```python
from build123d import *

# Parameters (mm, degrees)
SKETCH1_W           = 215
SKETCH1_H           = 14
BOSS_EXTRUDE1_DEPTH = 2
SKETCH2_W           = 215
SKETCH2_H           = 2
BOSS_EXTRUDE2_DEPTH = 4
SKETCH3_W           = 10
SKETCH3_H           = 10
BOSS_EXTRUDE3_DEPTH = 2
CUT_EXTRUDE1_DEPTH  = 4
BOSS_EXTRUDE4_START = -175
SKETCH8_W           = 10
SKETCH8_H           = 10
BOSS_EXTRUDE4_DEPTH = 50
CUT_EXTRUDE5_DEPTH  = 50
FILLET2_R           = 10
CUT_EXTRUDE6_DEPTH  = 10


with BuildPart() as part:
    # Sketch1 → Boss-Extrude1 (new body)
    with BuildSketch(Plane.XY):
        with Locations((-78.55, 1.825)):
            Rectangle(SKETCH1_W, SKETCH1_H)
    extrude(amount=BOSS_EXTRUDE1_DEPTH)

    # Sketch2 → Boss-Extrude2 (add)
    with BuildSketch(Plane.XY.offset(2)):
        with Locations((-78.55, -4.175)):
            Rectangle(SKETCH2_W, SKETCH2_H)
    extrude(amount=BOSS_EXTRUDE2_DEPTH)

    # Sketch3 → Boss-Extrude3 (add)
    with BuildSketch(Plane(origin=(0, 0, 0), x_dir=(-1, 0, 0), z_dir=(0, 0, -1))):
        with Locations((-33.95, 3.825)):
            Rectangle(SKETCH3_W, SKETCH3_H)
    extrude(amount=-BOSS_EXTRUDE3_DEPTH)

    # Sketch4 → Cut-Extrude1 (cut)
    with BuildSketch(Plane.XY.offset(6)):
        Polygon((28.95, -5.175), (8.95, -5.175), (3.95, -3.175), (28.95, -3.175), align=None)
    extrude(amount=-CUT_EXTRUDE1_DEPTH, mode=Mode.SUBTRACT)

    # Sketch8 → Boss-Extrude4 (add)
    with BuildSketch(Plane.ZY.offset(186.05).offset(BOSS_EXTRUDE4_START)):
        with Locations((7, 3.825)):
            Rectangle(SKETCH8_W, SKETCH8_H)
    extrude(amount=-BOSS_EXTRUDE4_DEPTH)

    # Sketch12 → Cut-Extrude5 (cut)
    with BuildSketch(Plane.XZ.offset(1.175)):
        Polygon((38.95, 0), (34.10168529, 12), (38.95, 12), align=None)
    extrude(amount=-CUT_EXTRUDE5_DEPTH, mode=Mode.SUBTRACT)

    # Fillet2
    fillet2_edges = [part.edges().sort_by_distance(p)[0] for p in [
        (36.525842645, 8.825, 6),
    ]]
    fillet(fillet2_edges, radius=FILLET2_R - 0.0001)  # a hair under: the kernel refuses the full size

    # Sketch13 → Cut-Extrude6 (cut)
    with BuildSketch(Plane.XY.offset(12)):
        with BuildLine():
            Line((-11.05, 8.825), (-11.05, -1.175))
            Line((-11.05, -1.175), (34.10168529, -1.175))
            add(Edge.make_bspline(
                [(-11.05, 8.825), (3.606248202, 7.334330419), (22.993995007, 11.334895317), (34.10168529, -1.175)],
                knots=[0, 0, 0, 0, 1, 1, 1, 1], degree=3))
        make_face()
    extrude(amount=-CUT_EXTRUDE6_DEPTH, mode=Mode.SUBTRACT)


solid = part.part
```
Verification items for the finished model (mm, model axes). A direction names the side the tool comes from. Coordinates: 2 decimals unless noted, no trailing zeros. Write each loop counter-clockwise with the first axis right and the second up, starting at its lowest first coordinate (ties: lowest second). Pieces come first, ordered by that corner, then holes. Notation, with made-up numbers: M 10.5,16 L 35.5,16 A22 cw 35.5,43 Z; hole C 6,-32 d2. An arc over 180 degrees is marked long. Answer as a JSON object with one key per item and string values. Group by question number.
(1) Cross-section at A-A, the plane x = -72.5. Record the cut outline in (y, z) (3 decimals), and give its area (3 significant figures).
(2) Tool access check on faces 1 (the face through (-30, 8.825, 1)), 2 (the face through (6.485, -4.189, 4.028)), 3 (the face through (34.3, -1.175, 3.3)). Record the directions out of +Z, -Z, +X, -X, +Y, -Y that give a thin tool (end or side, any length) a straight path to the whole face; none if there is none.
(3) Gauge pin test, flat ends, axial feed: pin 1 (7 mm diameter, centred on x = -88, y = 0, fed in from +Z); pin 2 (1.6 mm diameter, centred on y = -3, z = 1, fed in from +X); pin 3 (1 mm diameter, centred on y = -1.5, z = 3.5, fed in from -X); pin 4 (4.5 mm diameter, centred on x = -132.5, z = 3.5, fed in from +Y) (3 decimals). Record the tip position at first contact, or that the pin passes through.
(4) Material ranges on line 1 (Z direction, x = 23, y = 4.5); line 2 (Y direction, x = -119, z = 5) (3 decimals); line 3 (X direction, y = -0.25, z = 3.75), recorded low to high.
Reply:
{
 "1": {"outline": "M -5.175,0 L 8.825,0 L 8.825,2 L -3.175,2 L -3.175,6 L -5.175,6 Z", "area": "36.0 mm²"},
 "2": {"face 1": "+Z, -Z, +X, -X, +Y", "face 2": "+Z, +X", "face 3": "+Z, -Z, +X, -Y"},
 "3": {"pin 1": "z = 6", "pin 2": "x = 28.95", "pin 3": "x = 33.94", "pin 4": "y = 8.825"},
 "4": {"line 1": "0 to 2", "line 2": "-5.175 to -3.175", "line 3": "33.24 to 37.39"}
}
